Could you check a few things on this model? Use its own coordinates, in mm. A direction names the side the tool comes from. Coordinates: 2 decimals unless noted, no trailing zeros. Order: outer loops, then holes, each group sorted by start corner. A loop starts at its lowest first (then second) coordinate and runs counter-clockwise, first axis right, second up. Notation, with made-up numbers: M 33.25,66 L 39.25,66 A25 cw 39.25,85 Z; hole C -3.75,72.5 d5. An arc over 180 degrees is marked long. One line per question, with ' | ' between items. Start each with the question number.
from build123d import *

# Parameters (mm, degrees)
ESQUISSE2_R                  = 3
ENL_V_MAT_EXTRU_1_DEPTH      = 13.7
ESQUISSE3_R                  = 1.5
ENL_V_MAT_EXTRU_2_DEPTH      = 10
R_P_TITION_CIRCULAIRE1_COUNT = 4
ESQUISSE5_R                  = 2.5
ENL_V_MAT_EXTRU_3_DEPTH      = 12.05


with BuildPart() as part:
    # Esquisse1 → Révolution1 (revolve)
    with BuildSketch(Plane(origin=(0, 0, 0), x_dir=(1, 0, 0), z_dir=(0, 1, 0))):
        Polygon((-40.200130208, 0), (-40.200130208, 4.7), (-37.020130208, 4.7), (-37.020130208, 11.05), (-30.670130208, 11.05), (-30.670130208, 3.5), (-27.500130208, 3.5), (-27.500130208, 0), align=None)
    revolve(axis=Axis((-53.297005208, 0, 0), (1, 0, 0)))

    # Esquisse2 → Enlèv. mat.-Extru.1 (cut, through all)
    with BuildSketch(Plane.ZY.offset(40.200130208)):
        Circle(ESQUISSE2_R)
    extrude(amount=-ENL_V_MAT_EXTRU_1_DEPTH, mode=Mode.SUBTRACT)

    # Esquisse3 → Enlèv. mat.-Extru.2 (cut)
    with BuildSketch(Plane.ZY.offset(37.020130208)):
        with Locations((-5.656854249, 5.656854249)):
            Circle(ESQUISSE3_R)
    enl_v_mat_extru_2 = extrude(amount=-ENL_V_MAT_EXTRU_2_DEPTH, mode=Mode.SUBTRACT)

    # Répétition circulaire1: Enlèv. mat.-Extru.2 ×4 about axis
    r_p_tition_circulaire1_axis = Axis((0, 0, 0), (1, 0, 0))
    for i in range(1, R_P_TITION_CIRCULAIRE1_COUNT):
        add(enl_v_mat_extru_2.rotate(r_p_tition_circulaire1_axis, i * 360 / R_P_TITION_CIRCULAIRE1_COUNT), mode=Mode.SUBTRACT)

    # Esquisse5 → Enlèv. mat.-Extru.3 (cut, through all)
    with BuildSketch(Plane.XY):
        with Locations((-33.845130208, 0)):
            Circle(ESQUISSE5_R)
    extrude(amount=-ENL_V_MAT_EXTRU_3_DEPTH, mode=Mode.SUBTRACT)


solid = part.part
(1) Imagine slicing it at C-C, the plane z = -6.5. Write out the boundary of the cut face in (x, y), plus the area to 3 significant figures.
(2) Imagine slicing it at A-A, the plane y = 0. Write out the boundary of the cut face in (x, z).
(3) We'd pull the mould along Y, two halves only. Please class faces 4 (the cylindrical face through (-33.94, 0.9, 2.86)), 5 (the cylindrical face through (-29.063, -1.341, -3.233)), 6 (the flat face through (-37.02, -5, 0)): +Y half, -Y half, draft (parallel to the pull), parting line (faces both ways), or undercut.
(4) Imagine slicing it at D-D, the plane x = -31. Write out the boundary of the cut face in (y, z).
(5) If I drill on line 1 along Y through (x, z) = (-33.25, 0); line 2 along Y through (x, z) = (-36.5, -6.25); line 3 along Y through (x, z) = (-33.75, -7), over which ranges is the centre line in solid material (lowest first)? Write a range as from..to.
(6) For P1, Ø6, axis at y = 8, z = 4, coming from the +X side; P2, Ø6, axis at x = -38, y = -4.5, coming from the +Z side; P3, Ø3, axis at x = -31, z = -5, coming from the +Y side, each with a flat end and sliding along its axis, tell me the tip position at first contact or that it passes through.
(7) On a 3-axis mill with a long thin cutter (end or side, diameter ignored), from which of +Z, -Z, +X, -X, +Y, -Y can I reach the whole of each face in a straight line? I mean faces 1 (the cylindrical face through (-38.59, -4.59, 1.02)), 2 (the cylindrical face through (-32.692, -2.218, -6.288)), 3 (the flat face through (-30.67, 3, 3)). Say none if no direction works.
(8) Imagine slicing it at B-B, the plane z = 0. Write out the boundary of the cut face in (x, y), plus the area to 3 significant figures.
Answers:
1) outline: M -37.02,-8.94 L -30.67,-8.94 L -30.67,-6.9 L -37.02,-6.9 Z; M -37.02,-4.42 L -30.67,-4.42 L -30.67,4.42 L -37.02,4.42 Z; M -37.02,6.9 L -30.67,6.9 L -30.67,8.94 L -37.02,8.94 Z; hole C -33.85,0 d5 | area: 62.3 mm²
2) outline: M -40.2,-4.7 L -37.02,-4.7 L -37.02,-11.05 L -36.35,-11.05 L -36.35,-3 L -40.2,-3 Z; M -40.2,3 L -27.5,3 L -27.5,3.5 L -30.67,3.5 L -30.67,11.05 L -37.02,11.05 L -37.02,4.7 L -40.2,4.7 Z; M -31.35,-11.05 L -30.67,-11.05 L -30.67,-3.5 L -27.5,-3.5 L -27.5,-3 L -31.35,-3 Z
3) face 4: undercut | face 5: parting line | face 6: draft
4) outline: C 0,0 d22.1; hole C -5.66,-5.66 d3; hole C -5.66,5.66 d3; hole C 0,0 d6; hole C 5.66,-5.66 d3; hole C 5.66,5.66 d3
5) line 1: -11.05..-3, 3..11.05 | line 2: -9.11..-7.03, -4.28..4.28, 7.03..9.11 | line 3: -8.55..-6.32, -4.99..-2.5, 2.5..4.99, 6.32..8.55
6) P1: x = -30.67 | P2: z = 10.92 | P3: y = 10.48
7) face 1: -X | face 2: -Z | face 3: +X
8) outline: M -40.2,-4.7 L -37.02,-4.7 L -37.02,-11.05 L -30.67,-11.05 L -30.67,-3.5 L -27.5,-3.5 L -27.5,-3 L -40.2,-3 Z; M -40.2,3 L -27.5,3 L -27.5,3.5 L -30.67,3.5 L -30.67,11.05 L -37.02,11.05 L -37.02,4.7 L -40.2,4.7 Z | area: 116 mm²
